Source: three-view drawing plus pictorial views. Frame: mm from the lowest corner of the part. Coordinates: 2 decimals unless noted, no trailing zeros. Loops run counter-clockwise (first coordinate to the right, second up) from the corner with the lowest first, then second, coordinate; pieces in that order, holes last. Notation, with made-up numbers: (71.25, 10) - (99.25, 10) arc R23 ccw to (99.25, 31) - close; hole circle Ø3 at (-27.75, 16). An arc over 180 degrees is marked (long way). Return JSON: item names as keys, results as strings.
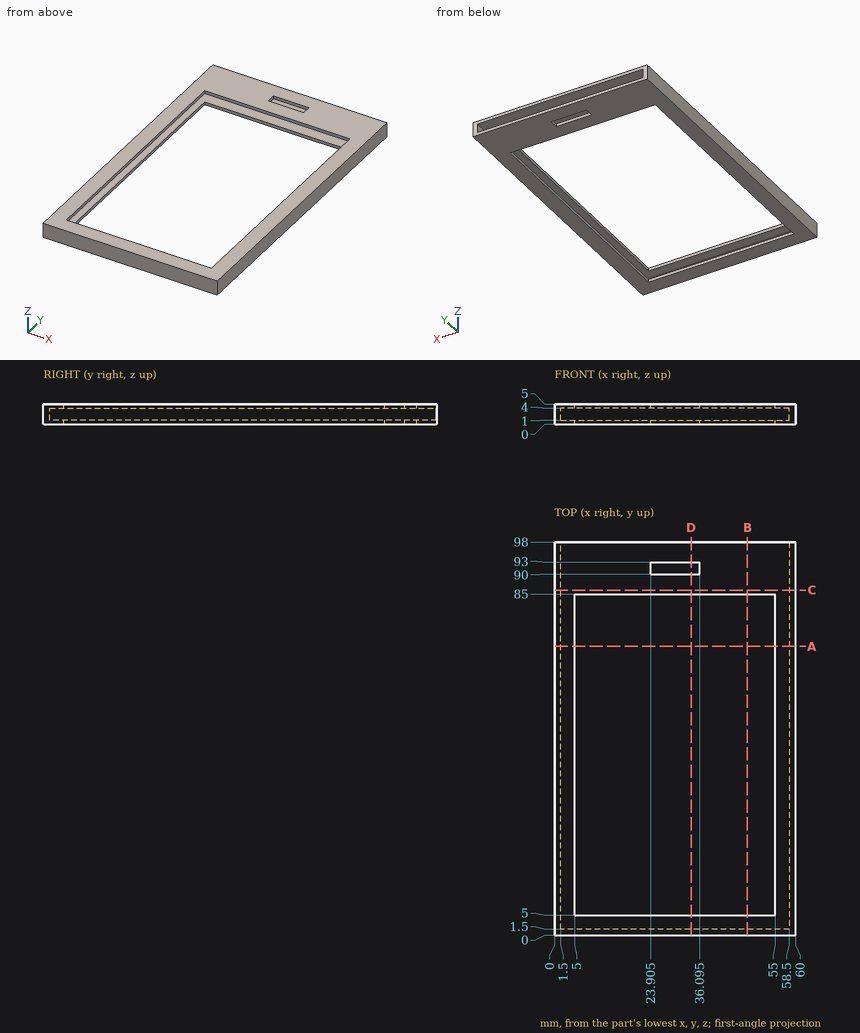
Item 1: First-contact query: pin 1 Ø8 at (x, y) = (47.5, 30.5) entering from -Z. Flat tip, straight axial feed; report the tip coordinate or a pass-through.
Worked out:
{"pin 1": "through"}
Item 2: Section query D-D, the plane x = 34. Return loops of the section in (y, z).
Worked out:
{"outline": "(0, 0) - (5, 0) - (5, 1) - (1.5, 1) - (1.5, 4) - (5, 4) - (5, 5) - (0, 5) - close; (85, 0) - (90, 0) - (90, 1) - (85, 1) - close; (85, 4) - (90, 4) - (90, 5) - (85, 5) - close; (93, 0) - (98, 0) - (98, 1) - (93, 1) - close; (93, 4) - (98, 4) - (98, 5) - (93, 5) - close"}
Item 3: Section query A-A, the plane y = 72. Return loops of the section in (x, z).
Worked out:
{"outline": "(0, 0) - (5, 0) - (5, 1) - (1.5, 1) - (1.5, 4) - (5, 4) - (5, 5) - (0, 5) - close; (55, 0) - (60, 0) - (60, 5) - (55, 5) - (55, 4) - (58.5, 4) - (58.5, 1) - (55, 1) - close"}
Item 4: Ray query, probe 1 along X at (y, z) = (20.5, 2.55); probe 2 along Z at (x, y) = (56, 32.5); probe 3 along Y at (x, z) = (44.5, 4.4). Return the intervals inside material, ascending. Write a range as from..to.
Worked out:
{"probe 1": "0..1.5, 58.5..60", "probe 2": "0..1, 4..5", "probe 3": "0..5, 85..98"}
Item 5: Section query B-B, the plane x = 48. Return loops of the section in (y, z).
Worked out:
{"outline": "(0, 0) - (5, 0) - (5, 1) - (1.5, 1) - (1.5, 4) - (5, 4) - (5, 5) - (0, 5) - close; (85, 0) - (98, 0) - (98, 1) - (85, 1) - close; (85, 4) - (98, 4) - (98, 5) - (85, 5) - close"}
Item 6: Section query C-C, the plane y = 86. Return loops of the section in (x, z), and give its area (3 significant figures).
Worked out:
{"outline": "(0, 0) - (60, 0) - (60, 5) - (0, 5) - close; hole (1.5, 1) - (58.5, 1) - (58.5, 4) - (1.5, 4) - close", "area": "129 mm^2"}
